Work out the finished part from the listing and answer in its coordinate system (mm). A direction names the side the tool comes from. Give positions to 0.01 mm unless a question says otherwise; leave off trailing zeros. Write each loop counter-clockwise with the first axis right and the second up, starting at its lowest first coordinate (ties: lowest second). Pieces come first, ordered by that corner, then holes. Notation, with made-up numbers: (81.25, -4) -> (129.25, -4) arc R35 cw to (129.25, 33) -> close; hole circle Ø3 at (68.5, 0.25). An arc over 180 degrees is marked (long way). Write item = value, one per line. Start each with the question number.
from build123d import *

# Parameters (mm, degrees)
F0_W      = 31.75
F0_H      = 60.198
F0_R      = 7.874
F1_DEPTH  = 10.922
F2_DEPTH  = 10.922
F3_W      = 10.922
F3_H      = 50.8
F4_DEPTH  = 33.528
F6_DEPTH  = 10.922
F7_W      = 33.528
F7_H      = 10.922
F8_DEPTH  = 52.578
F10_DEPTH = 10.922


with BuildPart() as f1:
    # F0 (on Front) → F1 (new body)
    with BuildSketch(Plane.XZ):
        with Locations((-44.894285, -4.041589)):
            Rectangle(F0_W, F0_H)
        Polygon((-29.019285, 26.057411), (-29.019285, -34.140589), (53.525416, -34.140589), (53.525416, 3.939625), align=None)
        with Locations((34.475416, -15.090589)):
            Circle(F0_R, mode=Mode.SUBTRACT)
    extrude(amount=F1_DEPTH)

    # F0 (on Front) → F2 (cut)
    with BuildSketch(Plane.XZ):
        with Locations((-44.894285, -4.041589)):
            Rectangle(F0_W, F0_H)
        Polygon((-29.019285, 26.057411), (-29.019285, -34.140589), (53.525416, -34.140589), (53.525416, 3.939625), align=None)
        with Locations((34.475416, -15.090589)):
            Circle(F0_R, mode=Mode.SUBTRACT)
    extrude(amount=-F2_DEPTH, mode=Mode.SUBTRACT)

    # F3 (on face) → F4 (join)
    with BuildSketch(Plane.XZ.offset(10.922)):
        with Locations((-55.308285, -8.740589)):
            Rectangle(F3_W, F3_H)
    extrude(amount=F4_DEPTH)

    # F5 (on face) → F6 (cut)
    with BuildSketch(Plane(origin=(-60.769285, 0, 0), x_dir=(0, -1, 0), z_dir=(-1, 0, 0))):
        Polygon((34.831685, 16.659411), (44.45, 0), (44.45, 16.659411), align=None)
    extrude(amount=-F6_DEPTH, mode=Mode.SUBTRACT)

    # F7 (on face) → F8 (join)
    with BuildSketch(Plane.YZ.offset(-49.847285)):
        with Locations((-27.686, -28.679589)):
            Rectangle(F7_W, F7_H)
    extrude(amount=F8_DEPTH)

    # F9 (on face) → F10 (cut)
    with BuildSketch(Plane.XY.offset(-23.218589)):
        Polygon((-14.706187, -10.922), (-49.847285, -33.637185), (-49.847285, -44.45), (2.730715, -44.45), (2.730715, -10.922), align=None)
    extrude(amount=-F10_DEPTH, mode=Mode.SUBTRACT)


solid = f1.part
(1) A cutting plane is placed at C-C, the plane z = -29. Write down the section's boundary in (x, y), then the cut area to 3 significant figures.
(2) Each of these flat-tipped pins is pushed along its axis until it touches: pin 1 (1.5 mm diameter, centred on y = -31, z = -12, fed in from +X); pin 2 (8.5 mm diameter, centred on x = -52.5, y = -20, fed in from +Z); pin 3 (9.5 mm diameter, centred on x = 34.48, z = -15.09, fed in from +Y); pin 4 (11.5 mm diameter, centred on x = -36, y = -25.5, fed in from +Z). Where does it stop, or does it pass through?
(3) A cutting plane is placed at D-D, the plane y = -21.5. Write down the section's boundary in (x, z), then the cut area to 3 significant figures.
(4) A cutting plane is placed at A-A, the plane z = -12. Write down the section's boundary in (x, y), then the cut area to 3 significant figures.
(5) Find the intervals of material crossed by line 1 along X through (y, z) = (-30, -22.5); line 2 along Y through (x, z) = (38.5, -4.5); line 3 along Z through (x, y) = (-50, -18.5), in increasing order.
(6) For faces 1 (the flat face through (-55, -44.45, -17)), 2 (the flat face through (-55, -23, 16.659)), 3 (the flat face through (-49.847, -27, -9)), determine the directions among +Z, -Z, +X, -X, +Y, -Y from which every point of the face is accessible in a straight line to the end or side of a thin tool.
(7) Determine the mould class of faces 4 (the cylindrical face through (41.749, -5.385, -18.106)), 5 (the flat face through (-32, -22.1, -28.6)), 6 (the flat face through (-45, -5, 26.057)) for opening direction Z: pulls with the +Z half, pulls with the -Z half, needs draft (parallel to the pull), parting line crosses it, or undercut.
(8) A cutting plane is placed at B-B, the plane x = 31. Write down the section's boundary in (y, z), then the cut area to 3 significant figures.
Results list:
q1.outline = (-60.77, -44.45) -> (-49.85, -44.45) -> (-49.85, -33.64) -> (-14.71, -10.92) -> (53.53, -10.92) -> (53.53, 0) -> (-60.77, 0) -> close
q1.area = 2,010 mm²
q2.pin_1 = -49.85
q2.pin_2 = 16.66
q2.pin_3 = through
q2.pin_4 = -23.22
q3.outline = (-60.77, -34.14) -> (-31.07, -34.14) -> (-31.07, -23.22) -> (-49.85, -23.22) -> (-49.85, 16.66) -> (-60.77, 16.66) -> close
q3.area = 760 mm²
q4.outline = (-60.77, -44.45) -> (-49.85, -44.45) -> (-49.85, -10.92) -> (27.23, -10.92) -> (27.23, 0) -> (-60.77, 0) -> close; (41.72, -10.92) -> (53.53, -10.92) -> (53.53, 0) -> (41.72, 0) -> close
q4.area = 1,460 mm²
q5.line_1 = -60.77 to -49.85
q5.line_2 = -10.92 to 0
q5.line_3 = -34.14 to 16.66
q6.face_1 = +Z, -Z, +X, -X, -Y
q6.face_2 = +Z, +X, -X, -Y
q6.face_3 = +Z, +X, -Y
q7.face_4 = undercut
q7.face_5 = needs draft
q7.face_6 = pulls with the +Z half
q8.outline = (-10.92, -34.14) -> (0, -34.14) -> (0, -22.16) -> (-10.92, -22.16) -> close; (-10.92, -8.03) -> (0, -8.03) -> (0, 9.98) -> (-10.92, 9.98) -> close
q8.area = 327 mm²
